```python
from build123d import *

# Parameters (mm, degrees)
ESQUISSE1_R             = 2
BOSS_EXTRU_2_DEPTH      = 5
ESQUISSE2_W             = 78
ESQUISSE2_H             = 23
ENL_V_MAT_EXTRU_2_DEPTH = 5


with BuildPart() as part:
    # Esquisse1 → Boss.-Extru.2 (new body)
    with BuildSketch(Plane.XY):
        with BuildLine():
            Line((0, 80), (-40.063357395, 80))
            Line((-40.063357395, 80), (-40.063357395, 43.608028339))
            Line((-40.063357395, 43.608028339), (-40.063357395, 23.347203835))
            Line((-40.063357395, 23.347203835), (-126.14466041, 23.347203835))
            Line((-126.14466041, 23.347203835), (-126.14466041, 43.608028339))
            Line((-126.14466041, 43.608028339), (-140.404811956, 43.608028339))
            ThreePointArc((-140.404811956, 43.608028339), (-170.122450923, 30.625328971), (-180.789117416, 0))
            ThreePointArc((-180.789117416, 0), (-170.122450923, -30.625328971), (-140.404811956, -43.608028339))
            Line((-140.404811956, -43.608028339), (-126.14466041, -43.608028339))
            Line((-126.14466041, -43.608028339), (-126.14466041, -23.347203835))
            Line((-126.14466041, -23.347203835), (-40.063357395, -23.347203835))
            Line((-40.063357395, -23.347203835), (-40.063357395, -43.608028339))
            Line((-40.063357395, -43.608028339), (-40.063357395, -80))
            Line((-40.063357395, -80), (0, -80))
            Line((0, -80), (0, 80))
        make_face()
        with Locations((-143.829395777, 36.206579824)):
            Circle(ESQUISSE1_R, mode=Mode.SUBTRACT)
        with Locations((-27.113068306, 36.206579824)):
            Circle(ESQUISSE1_R, mode=Mode.SUBTRACT)
        with Locations((-9.467128793, 72.29182392)):
            Circle(ESQUISSE1_R, mode=Mode.SUBTRACT)
        with Locations(Location((-9.538022857, -71.947546017, 0), (0, 0, 180))):
            Circle(ESQUISSE1_R, mode=Mode.SUBTRACT)
        with Locations(Location((-28.690315975, -37.022776214, 0), (0, 0, 180))):
            Circle(ESQUISSE1_R, mode=Mode.SUBTRACT)
        with Locations(Location((-143.994710805, -37.022776214, 0), (0, 0, 180))):
            Circle(ESQUISSE1_R, mode=Mode.SUBTRACT)
    extrude(amount=BOSS_EXTRU_2_DEPTH)

    # Esquisse2 → Enlèv. mat.-Extru.2 (cut)
    with BuildSketch(Plane.XY.offset(5)):
        with Locations((-107.776795965, 0)):
            Rectangle(ESQUISSE2_W, ESQUISSE2_H)
    extrude(amount=-ENL_V_MAT_EXTRU_2_DEPTH, mode=Mode.SUBTRACT)


solid = part.part
```
Here's how the part is built. I have some questions about the finished solid (model axes, mm). A direction names the side the tool comes from. Give positions to 0.01 mm unless a question says otherwise; leave off trailing zeros. Write each loop counter-clockwise with the first axis right and the second up, starting at its lowest first coordinate (ties: lowest second). Pieces come first, ordered by that corner, then holes. Notation, with made-up numbers: M 5,-36 L 52,-36 A26 cw 52,-14 Z; hole C -40,64 d9. An arc over 180 degrees is marked long. Put each result on its own line as item: value. Start each with the question number.
Item 1: Will these pins go through, and if not, where does the flat tip stop? pin 1 (1.5 mm diameter, centred on y = 59.5, z = 1.5, fed in from -X); pin 2 (2.5 mm diameter, centred on x = -28.69, y = -37.02, fed in from -Z); pin 3 (1.5 mm diameter, centred on x = -107.5, z = 2, fed in from -Y); pin 4 (3 mm diameter, centred on y = 12.5, z = 1, fed in from -X).
Item 2: If we section it at D-D, the plane x = -157.5: Write out the boundary of the cut face in (y, z), then the cut area to 3 significant figures.
Item 3: If we section it at C-C, the plane y = -53: Write out the boundary of the cut face in (x, z).
Item 4: Thinking about a two-plate mould opening in Y: for faces 4 (the flat face through (-20, 80, 2)), 5 (the flat face through (-84, -23.347, 2)), 6 (the cylindrical face through (-28.7, 34.99, 2.46)), which applies, +Y half, -Y half, draft (parallel to the pull), parting line (faces both ways), or undercut?
Item 5: If we section it at A-A, the plane x = -74: Write out the boundary of the cut face in (y, z).
Item 6: If we section it at B-B, the plane z = 0.9: Write out the boundary of the cut face in (x, y).
Item 7: On a 3-axis mill with a long thin cutter (end or side, diameter ignored), from which of +Z, -Z, +X, -X, +Y, -Y can I reach the whole of each face in a straight line? I mean faces 1 (the flat face through (-108, 11.5, 3)), 2 (the flat face through (-40.063, -51, 2)), 3 (the flat face through (-40.063, 52, 2)). Say none if no direction works.
Item 8: I need wall thicknesses on L1, parallel to Y at x = -121, z = 0.85; L2, parallel to X at y = -72, z = 2.3; L3, parallel to X at y = -2.5, z = 0.8. Which ranges of each line are inside material? Lowest first, please. Write a range as from..to.
Values:
1. pin 1: x = -40.06
1. pin 2: through
1. pin 3: y = -23.35
1. pin 4: x = -180.13
2. outline: M -39.82,0 L 39.82,0 L 39.82,5 L -39.82,5 Z
2. area: 398 mm²
3. outline: M -40.06,0 L 0,0 L 0,5 L -40.06,5 Z
4. face 4: +Y half
4. face 5: -Y half
4. face 6: undercut
5. outline: M -23.35,0 L -11.5,0 L -11.5,5 L -23.35,5 Z; M 11.5,0 L 23.35,0 L 23.35,5 L 11.5,5 Z
6. outline: M -180.79,0 A40.5 ccw -140.4,-43.61 L -126.14,-43.61 L -126.14,-23.35 L -40.06,-23.35 L -40.06,-80 L 0,-80 L 0,80 L -40.06,80 L -40.06,23.35 L -126.14,23.35 L -126.14,43.61 L -140.4,43.61 A40.5 ccw Z; hole M -146.78,-11.5 L -68.78,-11.5 L -68.78,11.5 L -146.78,11.5 Z; hole C -143.99,-37.02 d4; hole C -143.83,36.21 d4; hole C -28.69,-37.02 d4; hole C -27.11,36.21 d4; hole C -9.54,-71.95 d4; hole C -9.47,72.29 d4
7. face 1: +Z, -Z
7. face 2: +Z, -Z, -Y
7. face 3: +Z, -Z, +Y
8. L1: -23.35..-11.5, 11.5..23.35
8. L2: -40.06..-11.54, -7.54..0
8. L3: -180.9..-146.78, -68.78..0
